```python
from build123d import *

# Parameters (mm, degrees)
F0_R     = 38.1
F1_DEPTH = 50.8
F2_W     = 6.35
F2_H     = 6.35
F3_DEPTH = 76.2
F4_R     = 5.08
F5_SIZE  = 5.08


with BuildPart() as f1:
    # F0 (on Top) → F1 (new body)
    with BuildSketch(Plane.XY):
        Circle(F0_R)
    extrude(amount=F1_DEPTH)

    # F2 (on Top) → F3 (join)
    with BuildSketch(Plane.XY):
        with Locations((3.175, -3.723586)):
            Rectangle(F2_W, F2_H)
    extrude(amount=F3_DEPTH)

    # F4
    f4_edges = [f1.edges().sort_by_distance(p)[0] for p in [
        (-38.1, 0, 50.8),
    ]]
    fillet(f4_edges, radius=F4_R)

    # F5
    f5_edges = [f1.edges().sort_by_distance(p)[0] for p in [
        (6.35, -6.898586, 63.5),
        (-38.1, 0, 0),
    ]]
    chamfer(f5_edges, length=F5_SIZE)


solid = f1.part
```
For this review, take the finished solid that the model builds, in its own axes (mm). A direction names the side the tool comes from. Round coordinates to 2 decimals unless told otherwise and drop trailing zeros. Write each loop counter-clockwise with the first axis right and the second up, starting at its lowest first coordinate (ties: lowest second). Pieces come first, ordered by that corner, then holes. Notation, with made-up numbers: (-27.5, -39) - (-10.5, -39) arc R30 cw to (-10.5, -14) - close; hole circle Ø6 at (-30.5, 30.5). An arc over 180 degrees is marked (long way). Answer as CSV lines item,"result". Start each with the question number.
(1) Add section A-A, the plane z = 69. State the section outline as (x, y) points.
(2) Add section B-B, the plane z = 18. State the section outline as (x, y) points, plus the area to 3 significant figures.
(3) For line 1 (Z direction, x = 5.5, y = -19); line 2 (X direction, y = -0.5, z = 36); line 3 (Y direction, x = -9.5, z = 9), list the stretches that pass through material, from the lowest coordinate up.
(4) For pin 1 (3 mm diameter, centred on x = -25, y = 18, fed in from +Z); pin 2 (12 mm diameter, centred on y = -21.5, z = 39, fed in from -X); pin 3 (1 mm diameter, centred on x = 3.5, z = 8.5, fed in from -Y); pin 4 (10 mm diameter, centred on y = 3, z = 29.5, fed in from -X), all flat-tipped, find the tip position at first contact; note any pin that passes through.
(5) Machinability: for faces 1 (the flat face through (3.85, -4.32, 63.32)), 2 (the flat face through (3, -0.549, 63)), 3 (the flat face through (0, -4, 63)), 4 (the flat face through (0, 0, 0)), 5 (the conical face through (31.73, 9.992, 0.247)), which of the approach directions +Z, -Z, +X, -X, +Y, -Y give a long, thin tool a straight path to every point of the face, cutting with its end or side? Answer none if there is none.
From the geometry:
1,outline,"(0, -6.9) - (1.27, -6.9) - (6.35, -1.82) - (6.35, -0.55) - (0, -0.55) - close"
2,outline,"circle Ø76.2 at (0, 0)"
2,area,"4,560 mm²"
3,line 1,"z = 0 to 50.8"
3,line 2,"x = -38.1 to 38.1"
3,line 3,"y = -36.9 to 36.9"
4,pin 1,"stops at z = 50.8"
4,pin 2,"stops at x = -34.8"
4,pin 3,"stops at y = -37.98"
4,pin 4,"stops at x = -38.1"
5,face 1,"+Z, +X, -Y"
5,face 2,"+Z, +X, -X, +Y"
5,face 3,"+Z, -X, +Y, -Y"
5,face 4,"-Z, +X, -X, +Y, -Y"
5,face 5,"-Z"
